```python
from build123d import *

# Parameters (mm, degrees)
SZKIC2_R = 1.5


with BuildPart() as part:
    # Wyciągnięcie po ścieżce1: sweep along a path in Szkic1
    with BuildLine(Plane.XY) as wyci_gni_cie_po_cie_ce1_path:
        Line((60.5, -11.5), (0, -11.5))
        ThreePointArc((0, -11.5), (-10.250305385, 5.213563034), (9.294019694, 6.772827912))
        Line((9.294019694, 6.772827912), (14.754234774, -0.719957545))
        ThreePointArc((14.754234774, -0.719957545), (20.473785722, -4.243192601), (27.020890568, -2.739242316))
        ThreePointArc((27.020890568, -2.739242316), (32.983788023, -1.012326463), (38.740099231, -3.336819032))
        ThreePointArc((38.740099231, -3.336819032), (43.704455056, -5.474315656), (48.98666307, -4.328890373))
        Line((48.98666307, -4.328890373), (60.5, 2.318337803))
    # Szkic2 → Wyciągnięcie po ścieżce1 (sweep)
    with BuildSketch(Plane(origin=(60.5, -11.5, 0), x_dir=(0, 0, -1), z_dir=(1, 0, 0))):
        Circle(SZKIC2_R)
    sweep(path=wyci_gni_cie_po_cie_ce1_path.line)


solid = part.part
```
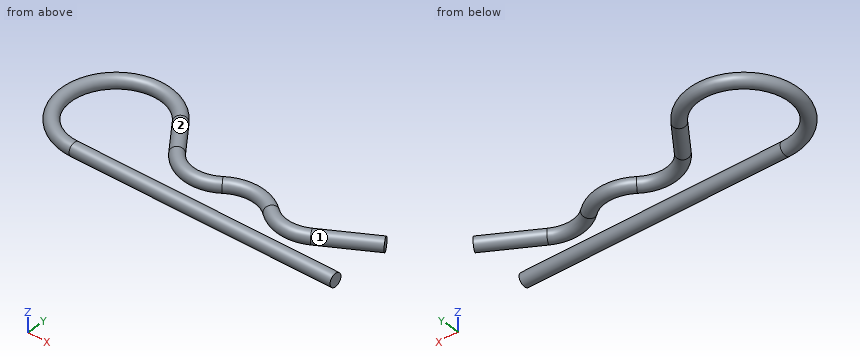
Source: CAD feature listing. Evaluate the final solid. Frame: model axes, mm. Face numbers are marked on the shaded views. Round coordinates to 2 decimals unless told otherwise and drop trailing zeros. Loops run counter-clockwise (first coordinate to the right, second up) from the corner with the lowest first, then second, coordinate; pieces in that order, holes last.
1. Contact query for flat-ended pins moving along their axis: pin 1 (0.9 mm diameter, centred on y = -11.5, z = -0.5, fed in from +X); pin 2 (1.5 mm diameter, centred on x = 36.5, z = 1, fed in from +Y); pin 3 (1 mm diameter, centred on x = 38.5, z = 0.5, fed in from +Y); pin 4 (5 mm diameter, centred on x = 10, y = 8, fed in from -Z). Output: stop coordinate, or through.
2. Section query A-A on z = -0.6. Output: boundary loops of the cut face in (x, y) (1 decimal), and give its area (3 significant figures).
3. Ray query, L1, parallel to X at y = -1.5, z = 0.85; L2, parallel to X at y = 5.25, z = -0.9; L3, parallel to Y at x = -5, z = 0.9 (3 decimals). Return the intervals inside material, ascending.
4. Mould query, pull axis Y, two halves, no side actions, for the marked faces 1 and 2. Classes: released by +Y, released by -Y, zero draft, split by the parting line, or undercut.
Answers below:
1. pin 1: stops at x = 60.5
1. pin 2: stops at y = -0.14
1. pin 3: stops at y = -1.03
1. pin 4: stops at z = -1.5
2. outline: (0, -12.9) - (60.5, -12.9) - (60.5, -10.1) - (0, -10.1) arc R10.1 cw (long way) to (8.2, 6) - (13.6, -1.5) arc R10.2 ccw to (27.8, -3.9) arc R8.1 cw to (37.8, -4.4) arc R10.2 ccw to (49.7, -5.5) - (61.2, 1.1) - (59.8, 3.5) - (48.3, -3.1) arc R7.5 cw to (39.6, -2.3) arc R10.9 ccw to (26.2, -1.6) arc R7.5 cw to (15.9, 0.1) - (10.4, 7.6) arc R12.9 ccw (long way) to start
2. area: 460 mm2
3. L1: x = -12.65 to -10.15, 13.79 to 17.21, 26.65 to 38.35, 51.41 to 56.36
3. L2: x = -11.56 to -8.86, 8.92 to 11.89
3. L3: y = -11.674 to -9.005, 9.005 to 11.674
4. face 1: undercut
4. face 2: undercut
